Input: part model. Units: mm. Frame: model coordinates. A direction names the side the tool comes from. Round coordinates to 2 decimals unless told otherwise and drop trailing zeros. Loops run counter-clockwise (first coordinate to the right, second up) from the corner with the lowest first, then second, coordinate; pieces in that order, holes last. Notation, with made-up numbers: M -17,-30 L 11,-30 A19 ccw 11,-23 Z; hole C 48.25,45 d11. An arc over 180 degrees is marked long. Return JSON: item names as keys, results as strings. Group by question number.
1) Material intervals for line 1 (X direction, y = 1.75, z = 42.5) (3 decimals); line 2 (X direction, y = 1, z = 39.5) (3 decimals); line 3 (Z direction, x = 45, y = 1.5), sorted ascending. Write a range as from..to.
2) Mould query, pull axis Z, two halves, no side actions, for faces 3 (the face through (-48, 1, 32)), 4 (the face through (-75.54, 1.01, -31.2)). Classes: +Z half, -Z half, draft (parallel to the pull), parting line (faces both ways), or undercut.
3) Section B-B (z = -31). Count the separate pieces of the cut face and the enclosed holes in it, plus the area to 3 significant figures.
4) Section C-C (x = 43.5). Output: boundary loops of the cut face in (y, z).
5) Section A-A (x = 60). Output: boundary loops of the cut face in (y, z).
6) Contact query for flat-ended pins moving along their axis: P1, Ø1, axis at y = 1.5, z = -3.5, coming from the +X side (3 decimals); P2, Ø1, axis at y = 1.5, z = 28, coming from the -X side (3 decimals); P3, Ø2.5, axis at x = 74.055, z = -31, coming from the +Y side. Output: stop coordinate, or through.
7) Access query for faces 1 (the face through (49, 1, 33)), 2 (the face through (60, 1, 39)). Directions: +Z, -Z, +X, -X, +Y, -Y. A direction counts if a zero-diameter tool reaches every point of the face in a straight line with its end or side. Return the directions, or none.
from build123d import *

# Parameters (mm, degrees)
SKETCH_1_W             = 139.61
SKETCH_1_H             = 92
EXTRUDE_1_DEPTH        = 2
SKETCH_2_W             = 40
SKETCH_2_H             = 2
SKETCH_2_W_2           = 15
EXTRUDE_2_DEPTH        = 3
SKETCH_3_W             = 20
SKETCH_3_H             = 2
EXTRUDE_3_DEPTH        = 7
SKETCH_4_R             = 1.5
CUT_EXTRUDE_1_DEPTH    = 92.126330031
CUT_EXTRUDE_2_DEPTH    = 92.126330031
PATTERN_LINEAR_1_COUNT = 9
PATTERN_LINEAR_1_PITCH = 15
SKETCH_8_R             = 1.5
CUT_EXTRUDE_4_DEPTH    = 92.126330031
SKETCH_10_W            = 25
SKETCH_10_H            = 5
EXTRUDE_5_DEPTH        = 2
SKETCH_12_W            = 25
SKETCH_12_H            = 15
CUT_EXTRUDE_5_DEPTH    = 92.126330031
FILLET_1_R             = 5
CUT_EXTRUDE_6_DEPTH    = 92.126330031
EXTRUDE_6_DEPTH        = 2
FILLET_2_R             = 5
SKETCH_15_W            = 3
SKETCH_15_H            = 20
EXTRUDE_7_DEPTH        = 2


with BuildPart() as part:
    # 草图1 → 凸台-拉伸1 (new body)
    with BuildSketch(Plane(origin=(0, 0, 0), x_dir=(1, 0, 0), z_dir=(0, 1, 0))):
        Rectangle(SKETCH_1_W, SKETCH_1_H)
    extrude(amount=EXTRUDE_1_DEPTH)

    # 草图2 → 凸台-拉伸2 (add)
    with BuildSketch(Plane.XY.offset(46)):
        with Locations((0, 1)):
            Rectangle(SKETCH_2_W, SKETCH_2_H)
        with Locations((57.5, 1)):
            Rectangle(SKETCH_2_W_2, SKETCH_2_H)
        with Locations((-57.5, 1)):
            Rectangle(SKETCH_2_W_2, SKETCH_2_H)
    extrude(amount=EXTRUDE_2_DEPTH)

    # 草图3 → 凸台-拉伸3 (add)
    with BuildSketch(Plane(origin=(69.805, 0, 0), x_dir=(0, 0, -1), z_dir=(1, 0, 0))):
        with Locations((31, 1)):
            Rectangle(SKETCH_3_W, SKETCH_3_H)
    extrude_3 = extrude(amount=EXTRUDE_3_DEPTH)

    # 草图4 → 切除-拉伸1 (cut, through all)
    with BuildSketch(Plane(origin=(0, 2, 0), x_dir=(1, 0, 0), z_dir=(0, 1, 0))):
        with Locations(Location((74.055, 31, 0), (0, 0, 270))):
            Circle(SKETCH_4_R)
    cut_extrude_1 = extrude(amount=-CUT_EXTRUDE_1_DEPTH, mode=Mode.SUBTRACT)

    # 草图5 → 切除-拉伸2 (cut, through all)
    with BuildSketch(Plane(origin=(0, 2, 0), x_dir=(1, 0, 0), z_dir=(0, 1, 0))):
        with BuildLine():
            Line((-65, -34), (-65, 34))
            ThreePointArc((-65, 34), (-60, 39), (-55, 34))
            Line((-55, 34), (-55, -34))
            ThreePointArc((-55, -34), (-60, -39), (-65, -34))
        make_face()
    cut_extrude_2 = extrude(amount=-CUT_EXTRUDE_2_DEPTH, mode=Mode.SUBTRACT)

    # 阵列(线性)1: 切除-拉伸2 ×9
    with Locations(*[(i * PATTERN_LINEAR_1_PITCH, 0, 0) for i in range(1, PATTERN_LINEAR_1_COUNT)]):
        add(cut_extrude_2, mode=Mode.SUBTRACT)

    # 草图8 → 切除-拉伸4 (cut, through all)
    with BuildSketch(Plane.XZ):
        with Locations(Location((52.5, -42, 0), (0, 0, 270))):
            Circle(SKETCH_8_R)
    cut_extrude_4 = extrude(amount=-CUT_EXTRUDE_4_DEPTH, mode=Mode.SUBTRACT)

    # 镜向4: 切除-拉伸4 across plane
    add(cut_extrude_4.mirror(Plane(origin=(0, 0, 0), x_dir=(0, 0, 1), z_dir=(1, 0, 0))), mode=Mode.SUBTRACT)

    # 草图10 → 凸台-拉伸5 (add)
    with BuildSketch(Plane(origin=(0, 2, 0), x_dir=(1, 0, 0), z_dir=(0, 1, 0))):
        with Locations((37.5, -31.5)):
            Rectangle(SKETCH_10_W, SKETCH_10_H)
        with Locations((-37.5, -31.5)):
            Rectangle(SKETCH_10_W, SKETCH_10_H)
    extrude(amount=-EXTRUDE_5_DEPTH)

    # 草图12 → 切除-拉伸5 (cut, through all)
    with BuildSketch(Plane(origin=(0, 2, 0), x_dir=(1, 0, 0), z_dir=(0, 1, 0))):
        with Locations((-37.5, -38.5)):
            Rectangle(SKETCH_12_W, SKETCH_12_H)
        with Locations((37.5, -38.5)):
            Rectangle(SKETCH_12_W, SKETCH_12_H)
    extrude(amount=-CUT_EXTRUDE_5_DEPTH, mode=Mode.SUBTRACT)

    # 圆角1
    fillet_1_edges = [part.edges().sort_by_distance(p)[0] for p in [
        (-40, 1, 29),
        (-50, 1, 29),
        (-25, 1, 31),
        (-50, 1, 31),
        (50, 1, 31),
        (25, 1, 31),
        (50, 1, 29),
        (40, 1, 29),
        (35, 1, 29),
        (25, 1, 29),
        (-25, 1, 29),
        (-35, 1, 29),
    ]]
    fillet(fillet_1_edges, radius=FILLET_1_R - 0.0001)  # a hair under: the kernel refuses the full size

    # 草图13 → 切除-拉伸6 (cut, through all)
    with BuildSketch(Plane(origin=(0, 2, 0), x_dir=(1, 0, 0), z_dir=(0, 1, 0))):
        with BuildLine():
            Line((-10, 7), (10, 7))
            ThreePointArc((10, 7), (15, 2), (10, -3))
            Line((10, -3), (-10, -3))
            ThreePointArc((-10, -3), (-15, 2), (-10, 7))
        make_face()
    extrude(amount=-CUT_EXTRUDE_6_DEPTH, mode=Mode.SUBTRACT)

    # 草图14 → 凸台-拉伸6 (add)
    with BuildSketch(Plane(origin=(0, 2, 0), x_dir=(1, 0, 0), z_dir=(0, 1, 0))):
        Polygon((20, 7), (2.5, 7), (2.5, -3), (20, -3), (20, -8), (-20, -8), (-20, -3), (-2.5, -3), (-2.5, 7), (-20, 7), (-20, 12), (20, 12), align=None)
    extrude(amount=-EXTRUDE_6_DEPTH)

    # 圆角2
    fillet_2_edges = [part.edges().sort_by_distance(p)[0] for p in [
        (-10, 1, -12),
        (-20, 1, -12),
        (-5, 1, -12),
        (5, 1, -12),
        (10, 1, -12),
        (20, 1, -12),
        (20, 1, 3),
        (20, 1, -7),
        (20, 1, 8),
        (10, 1, 8),
        (-5, 1, 8),
        (5, 1, 8),
        (-10, 1, 8),
        (-20, 1, 8),
        (2.5, 1, 3),
        (2.5, 1, -7),
        (-2.5, 1, 3),
        (-2.5, 1, -7),
        (-20, 1, 3),
        (-20, 1, -7),
    ]]
    fillet(fillet_2_edges, radius=FILLET_2_R - 0.0001)  # a hair under: the kernel refuses the full size

    # 镜向5: 凸台-拉伸3, 切除-拉伸1 across plane
    add(extrude_3.mirror(Plane(origin=(0, 0, 0), x_dir=(0, 0, 1), z_dir=(1, 0, 0))))
    add(cut_extrude_1.mirror(Plane(origin=(0, 0, 0), x_dir=(0, 0, 1), z_dir=(1, 0, 0))), mode=Mode.SUBTRACT)

    # 草图15 → 凸台-拉伸7 (add)
    with BuildSketch(Plane(origin=(0, 2, 0), x_dir=(1, 0, 0), z_dir=(0, 1, 0))):
        with Locations((71.305, -31)):
            Rectangle(SKETCH_15_W, SKETCH_15_H)
        with Locations((-71.305, -31)):
            Rectangle(SKETCH_15_W, SKETCH_15_H)
    extrude(amount=-EXTRUDE_7_DEPTH)


solid = part.part
Returned:
{
 "1": {"line 1": "x = -69.805..-50, -25..25, 50..69.805", "line 2": "x = -72.805..-50, -25..25, 50..72.805", "line 3": "z = -46..-39, 29..31"},
 "2": {"face 3": "+Z half", "face 4": "undercut"},
 "3": {"separate pieces": "12", "enclosed holes": "0", "area": "115 mm^2"},
 "4": {"outline": "M 0,-46 L 2,-46 L 2,-38.77 L 0,-38.77 Z; M 0,28.77 L 2,28.77 L 2,31 L 0,31 Z"},
 "5": {"outline": "M 0,-46 L 2,-46 L 2,-39 L 0,-39 Z; M 0,39 L 2,39 L 2,49 L 0,49 Z"},
 "6": {"P1": "stops at x = 69.805", "P2": "stops at x = -72.805", "P3": "passes through"},
 "7": {"face 1": "+Z, +Y, -Y", "face 2": "+Y, -Y"}
}
